```python
from build123d import *

# Parameters (mm, degrees)
PAD_DEPTH       = 20
SKETCH006_R     = 10
POCKET_DEPTH    = 20.001
SKETCH005_R     = 11.05
POCKET001_DEPTH = 7
SKETCH002_R     = 2.25
POCKET002_DEPTH = 50.001
SKETCH009_R     = 11.05
POCKET006_DEPTH = 7
SKETCH010_R     = 6.05
POCKET007_DEPTH = 20.001
SKETCH011_W     = 25
SKETCH011_H     = 1
POCKET008_DEPTH = 20.001
SKETCH012_R     = 1.25
POCKET009_DEPTH = 20.001
SKETCH008_R     = 5
POCKET010_DEPTH = 5
SKETCH013_R     = 5
POCKET011_DEPTH = 5
SKETCH014_R     = 5
POCKET012_DEPTH = 5
POCKET013_DEPTH = 15
SKETCH016_R     = 1.25
POCKET014_DEPTH = 20.001
SKETCH017_R     = 3
POCKET015_DEPTH = 3
SKETCH018_R     = 12
POCKET016_DEPTH = 5
FILLET_R        = 9


with BuildPart() as part:
    # Sketch → Pad (new body)
    with BuildSketch(Plane.XY):
        with BuildLine():
            Line((-53.330303, 22), (95, 22))
            Line((95, 12.5), (95, 22))
            Line((95, 12.5), (80, 12.5))
            Line((80, -28), (80, 12.5))
            Line((28, -28), (80, -28))
            Line((28, -28), (28, -12.639225))
            Line((28, -12.639225), (15.5, -12.639225))
            ThreePointArc((-18.330303, -8), (-2.717215, -19.814559), (15.5, -12.639225))
            Line((-18.330303, -8), (-53.330303, -8))
            Line((-53.330303, -8), (-53.330303, 22))
        make_face()
    extrude(amount=PAD_DEPTH)

    # Sketch006 → Pocket (cut, through all)
    with BuildSketch(Plane(origin=(0, 0, 0), x_dir=(1, 0, 0), z_dir=(0, 0, -1))):
        Circle(SKETCH006_R)
    extrude(amount=-POCKET_DEPTH, mode=Mode.SUBTRACT)

    # Sketch005 → Pocket001 (cut)
    with BuildSketch(Plane.XY.offset(20)):
        Circle(SKETCH005_R)
    extrude(amount=-POCKET001_DEPTH, mode=Mode.SUBTRACT)

    # Sketch002 → Pocket002 (cut, through all)
    with BuildSketch(Plane.XZ.offset(28)):
        with Locations((21.75, 10)):
            Circle(SKETCH002_R)
        with Locations((-45, 10)):
            Circle(SKETCH002_R)
        with Locations((87, 10)):
            Circle(SKETCH002_R)
    extrude(amount=-POCKET002_DEPTH, mode=Mode.SUBTRACT)

    # Sketch009 → Pocket006 (cut)
    with BuildSketch(Plane(origin=(0, 0, 0), x_dir=(1, 0, 0), z_dir=(0, 0, -1))):
        Circle(SKETCH009_R)
    extrude(amount=-POCKET006_DEPTH, mode=Mode.SUBTRACT)

    # Sketch010 → Pocket007 (cut, through all)
    with BuildSketch(Plane.XY.offset(20)):
        with Locations((-35, 5)):
            Circle(SKETCH010_R)
    extrude(amount=-POCKET007_DEPTH, mode=Mode.SUBTRACT)

    # Sketch011 → Pocket008 (cut, through all)
    with BuildSketch(Plane.XY.offset(20)):
        with Locations((-42.5, 4.75)):
            Rectangle(SKETCH011_W, SKETCH011_H)
    extrude(amount=-POCKET008_DEPTH, mode=Mode.SUBTRACT)

    # Sketch012 → Pocket009 (cut, through all)
    with BuildSketch(Plane.XY.offset(20)):
        with Locations((11.691343, 6.75)):
            Circle(SKETCH012_R)
        with Locations((-11.691343, 6.75)):
            Circle(SKETCH012_R)
        with Locations((0, -13.5)):
            Circle(SKETCH012_R)
    extrude(amount=-POCKET009_DEPTH, mode=Mode.SUBTRACT)

    # Sketch008 → Pocket010 (cut)
    with BuildSketch(Plane.XZ.offset(8)):
        with Locations((-45, 10)):
            Circle(SKETCH008_R)
    extrude(amount=-POCKET010_DEPTH, mode=Mode.SUBTRACT)

    # Sketch013 → Pocket011 (cut)
    with BuildSketch(Plane.XZ.offset(12.639225)):
        with Locations((21.75, 10)):
            Circle(SKETCH013_R)
    extrude(amount=-POCKET011_DEPTH, mode=Mode.SUBTRACT)

    # Sketch014 → Pocket012 (cut)
    with BuildSketch(Plane.XZ.offset(-12.5)):
        with Locations((87, 10)):
            Circle(SKETCH014_R)
    extrude(amount=-POCKET012_DEPTH, mode=Mode.SUBTRACT)

    # Sketch015 → Pocket013 (cut)
    with BuildSketch(Plane.XY.offset(20)):
        Polygon((31.25, -19.5), (31.25, 15.5), (36.199747, 20.449747), (71.199747, 20.449747), (76.149495, 15.5), (76.149495, -19.5), (71.199747, -24.449747), (36.199747, -24.449747), align=None)
    extrude(amount=-POCKET013_DEPTH, mode=Mode.SUBTRACT)

    # Sketch016 → Pocket014 (cut, through all)
    with BuildSketch(Plane(origin=(0, 0, 0), x_dir=(1, 0, 0), z_dir=(0, 0, -1))):
        with Locations((38.25, 17.5)):
            Circle(SKETCH016_R)
        with Locations((69.25, 17.5)):
            Circle(SKETCH016_R)
        with Locations((38.25, -13.5)):
            Circle(SKETCH016_R)
        with Locations((69.25, -13.5)):
            Circle(SKETCH016_R)
    extrude(amount=-POCKET014_DEPTH, mode=Mode.SUBTRACT)

    # Sketch017 → Pocket015 (cut)
    with BuildSketch(Plane(origin=(0, 0, 0), x_dir=(1, 0, 0), z_dir=(0, 0, -1))):
        with Locations((38.25, 17.5)):
            Circle(SKETCH017_R)
        with Locations((69.25, 17.5)):
            Circle(SKETCH017_R)
        with Locations((38.25, -13.5)):
            Circle(SKETCH017_R)
        with Locations((69.25, -13.5)):
            Circle(SKETCH017_R)
    extrude(amount=-POCKET015_DEPTH, mode=Mode.SUBTRACT)

    # Sketch018 → Pocket016 (cut)
    with BuildSketch(Plane(origin=(0, 0, 0), x_dir=(1, 0, 0), z_dir=(0, 0, -1))):
        with Locations((53.75, 2)):
            Circle(SKETCH018_R)
    extrude(amount=-POCKET016_DEPTH, mode=Mode.SUBTRACT)

    # Fillet
    fillet_edges = [part.edges().sort_by_distance(p)[0] for p in [
        (28, -28, 10),
        (80, -28, 10),
    ]]
    fillet(fillet_edges, radius=FILLET_R)


solid = part.part
```
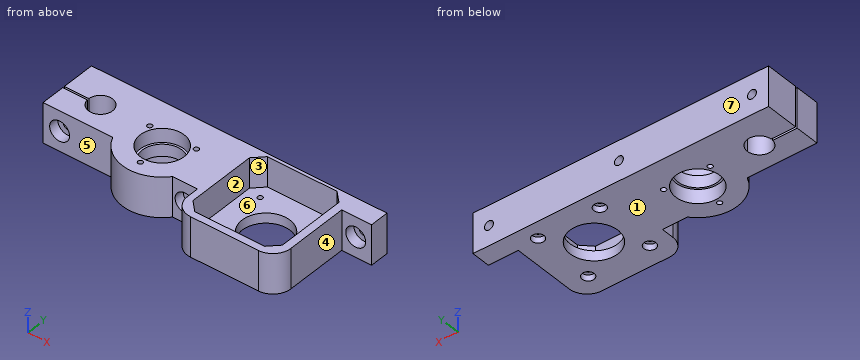
Check sheet for the modelled part. Datum: model origin and axes. Units: mm. Face numbers are marked on the shaded views. A direction names the side the tool comes from. Round coordinates to 2 decimals unless told otherwise and drop trailing zeros. Order: outer loops, then holes, each group sorted by start corner. A loop starts at its lowest first (then second) coordinate and runs counter-clockwise, first axis right, second up. Notation, with made-up numbers: (-2, 65) -> (47, 65) arc R31 cw to (47, 94) -> close; hole circle Ø9 at (19.25, 80). An arc over 180 degrees is marked (long way). Use CSV: the item, a comma, the result in double quotes.
(1) Depth check by flat-ended pin: pin 1 (3 mm diameter, centred on x = 20.5, z = 9, fed in from -Y); pin 2 (2.5 mm diameter, centred on x = -45, z = 10, fed in from +Y); pin 3 (7 mm diameter, centred on x = 38.25, y = -17.5, fed in from +Z); pin 4 (10 mm diameter, centred on y = -18.5, z = 12.5, fed in from -X). Enter the tip coordinate at first touch or a pass-through.
Worked out:
pin 1,"y = -7.64"
pin 2,"through"
pin 3,"z = 5"
pin 4,"x = -14.76"
(2) Cross-section at B-B (z = 17.25). Record the boundary of the cut face in (x, y).
Worked out:
outline,"(-53.33, -8) -> (-18.33, -8) arc R20 ccw to (15.5, -12.64) -> (28, -12.64) -> (28, -19) arc R9 ccw to (37, -28) -> (71, -28) arc R9 ccw to (80, -19) -> (80, 12.5) -> (95, 12.5) -> (95, 22) -> (-53.33, 22) -> (-53.33, 5.25) -> (-41.04, 5.25) arc R6.05 cw (long way) to (-41, 4.25) -> (-53.33, 4.25) -> close; hole circle Ø2.5 at (-11.69, 6.75); hole circle Ø22.1 at (0, 0); hole circle Ø2.5 at (0, -13.5); hole circle Ø2.5 at (11.69, 6.75); hole (31.25, -19.5) -> (36.2, -24.45) -> (71.2, -24.45) -> (76.15, -19.5) -> (76.15, 15.5) -> (71.2, 20.45) -> (36.2, 20.45) -> (31.25, 15.5) -> close"
(3) Material ranges on line 1 along X through (y, z) = (13.5, 4.4); line 2 along Y through (x, z) = (0, 8.95); line 3 along Y through (x, z) = (69.25, 3.95), recorded low to high. Write a range as from..to.
Worked out:
line 1,"-53.33..37, 39.5..68, 70.5..95"
line 2,"-20..-14.75, -12.25..-10, 10..22"
line 3,"-28..-18.75, -16.25..12.25, 14.75..22"
(4) Draft check along X on the marked faces 1, 2, 3 and 4. Enter one of: pulls with the +X half, pulls with the -X half, needs draft (parallel to the pull), parting line crosses it, or undercut.
Worked out:
face 1,"needs draft"
face 2,"undercut"
face 3,"undercut"
face 4,"pulls with the +X half"
(5) Cross-section at C-C (z = 10). Count the separate pieces of the cut face and the enclosed holes in it, and give its area (3 significant figures).
Worked out:
separate pieces,"5"
enclosed holes,"5"
area,"2,680 mm²"
(6) Cross-section at A-A (x = -35). Record the boundary of the cut face in (y, z), and give its area (3 significant figures).
Worked out:
outline,"(-8, 0) -> (-1.05, 0) -> (-1.05, 20) -> (-8, 20) -> close; (11.05, 0) -> (22, 0) -> (22, 20) -> (11.05, 20) -> close"
area,"358 mm²"
(7) Cross-section at D-D (x = 61.5). Record the boundary of the cut face in (y, z), and give its area (3 significant figures).
Worked out:
outline,"(-28, 0) -> (-11.16, 0) -> (-11.16, 5) -> (-24.45, 5) -> (-24.45, 20) -> (-28, 20) -> close; (7.16, 0) -> (22, 0) -> (22, 20) -> (20.45, 20) -> (20.45, 5) -> (7.16, 5) -> close"
area,"235 mm²"
(8) Tool access check on the marked faces 5, 6 and 7. Record the directions out of +Z, -Z, +X, -X, +Y, -Y that give a thin tool (end or side, any length) a straight path to the whole face; none if there is none.
Worked out:
face 5,"+Z, -Z, -X, -Y"
face 6,"+Z"
face 7,"+Z, -Z, +X, -X, +Y"
